For this review, take the finished solid that the model builds, in its own axes (mm). Give positions to 0.01 mm unless a question says otherwise; leave off trailing zeros. Write each loop counter-clockwise with the first axis right and the second up, starting at its lowest first coordinate (ties: lowest second). Pieces come first, ordered by that corner, then holes. Notation, with made-up numbers: M 72,66.25 L 103,66.25 A23 ccw 103,80.25 Z; hole C 68.5,89 d11. An arc over 180 degrees is marked long. One line per item, written item: value. Start each with the question number.
Item 1: Clearance check with flat-ended pins moving along their axes: pin 1 Ø2 at (y, z) = (-33, 12.5) entering from -X; pin 2 Ø7 at (x, y) = (507, -30.5) entering from +Z; pin 3 Ø3 at (y, z) = (-30, 14.5) entering from +X. State where each tip first meets the part, or that it passes through.
Item 2: To check wall thickness, follow probe 1 along Y at (x, z) = (339, 10.5); probe 2 along Y at (x, z) = (-170, 15.75); probe 3 along Z at (x, y) = (128.5, -19). State the ranges of each line that lie inside material, in increasing order.
Item 3: Consider section A-A, the plane z = 11.75. Write out the cut boundary in (x, y).
Item 4: Consider section B-B, the plane x = 458.5. Write out the cut boundary in (y, z).
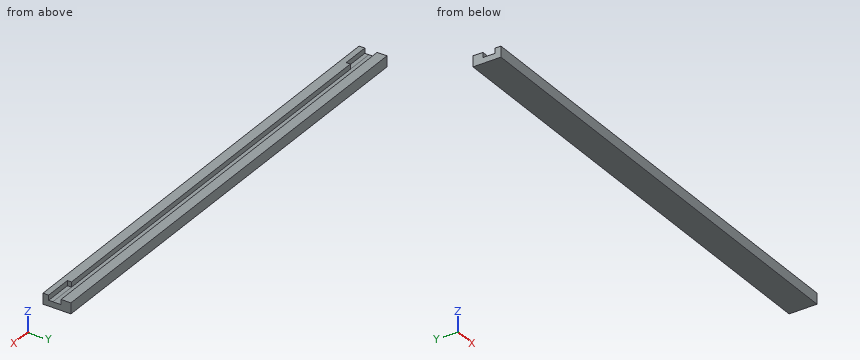
```python
from build123d import *

# Parameters (mm, degrees)
F0_W     = 745
F0_H     = 44
F1_DEPTH = 17
F2_W     = 12.964161098
F2_H     = 8.0115068778
F3_DEPTH = 745
F4_W     = 44
F4_H     = 6.5
F5_DEPTH = 8
F6_W     = 44
F6_H     = 6.5
F7_DEPTH = 8


with BuildPart() as f1:
    # F0 (on Top) → F1 (new body)
    with BuildSketch(Plane.XY):
        with Locations((164.9187269809, -22)):
            Rectangle(F0_W, F0_H)
    extrude(amount=F1_DEPTH)

    # F2 (on face) → F3 (cut)
    with BuildSketch(Plane.YZ.offset(537.4187269809)):
        with Locations((-22.017919451, 12.9942465611)):
            Rectangle(F2_W, F2_H)
    extrude(amount=-F3_DEPTH, mode=Mode.SUBTRACT)

    # F4 (on face) → F5 (cut)
    with BuildSketch(Plane.XY.offset(17)):
        with Locations((515.4187269809, -31.75)):
            Rectangle(F4_W, F4_H)
    extrude(amount=-F5_DEPTH, mode=Mode.SUBTRACT)

    # F6 (on face) → F7 (cut)
    with BuildSketch(Plane.XY.offset(17)):
        with Locations((-185.5812730191, -31.75)):
            Rectangle(F6_W, F6_H)
    extrude(amount=-F7_DEPTH, mode=Mode.SUBTRACT)


solid = f1.part
```
Model answer:
1. pin 1: stops at x = -163.58
1. pin 2: stops at z = 9
1. pin 3: stops at x = 493.42
2. probe 1: y = -44 to -28.5, -15.54 to 0
2. probe 2: y = -44 to -35, -15.54 to 0
2. probe 3: z = 0 to 8.99
3. outline: M -207.58,-44 L 537.42,-44 L 537.42,-35 L 493.42,-35 L 493.42,-28.5 L -163.58,-28.5 L -163.58,-35 L -207.58,-35 Z; M -207.58,-15.54 L 537.42,-15.54 L 537.42,0 L -207.58,0 Z
4. outline: M -44,0 L 0,0 L 0,17 L -15.54,17 L -15.54,8.99 L -28.5,8.99 L -28.5,17 L -44,17 Z
